Part model, mm, in its own coordinate system. A direction names the side the tool comes from. Give positions to 0.01 mm unless a question says otherwise; leave off trailing zeros. Order: outer loops, then holes, each group sorted by start corner. A loop starts at its lowest first (then second) coordinate and runs counter-clockwise, first axis right, second up. Notation, with made-up numbers: M -11.5,88.5 L 20.5,88.5 A18 cw 20.5,121.5 Z; hole C -38,-7.5 d4. An arc over 180 degrees is marked long. Return JSON: item names as keys, results as strings.
from build123d import *

# Parameters (mm, degrees)
SKETCH1_W           = 45
SKETCH1_H           = 55
BOSS_EXTRUDE1_DEPTH = 165
BOSS_EXTRUDE2_DEPTH = 75
SKETCH3_W           = 205
SKETCH3_H           = 80
CUT_EXTRUDE1_DEPTH  = 5
SKETCH4_W           = 205
SKETCH4_H           = 70
CUT_EXTRUDE2_DEPTH  = 15


with BuildPart() as part:
    # Sketch1 → Boss-Extrude1 (new body)
    with BuildSketch(Plane.XY):
        with Locations((22.5, 27.5)):
            Rectangle(SKETCH1_W, SKETCH1_H)
    extrude(amount=BOSS_EXTRUDE1_DEPTH)

    # Sketch2 → Boss-Extrude2 (add)
    with BuildSketch(Plane(origin=(0, 0, 0), x_dir=(-1, 0, 0), z_dir=(0, 0, -1))):
        Polygon((0, 0), (80, 0), (80, 80), (-125, 80), (-125, 0), (-45, 0), align=None)
    extrude(amount=-BOSS_EXTRUDE2_DEPTH)

    # Sketch3 → Cut-Extrude1 (cut)
    with BuildSketch(Plane(origin=(0, 0, 0), x_dir=(-1, 0, 0), z_dir=(0, 0, -1))):
        with Locations((-22.5, 40)):
            Rectangle(SKETCH3_W, SKETCH3_H)
    extrude(amount=-CUT_EXTRUDE1_DEPTH, mode=Mode.SUBTRACT)

    # Sketch4 → Cut-Extrude2 (cut)
    with BuildSketch(Plane(origin=(0, 80, 0), x_dir=(1, 0, 0), z_dir=(0, 1, 0))):
        with Locations((22.5, -40)):
            Rectangle(SKETCH4_W, SKETCH4_H)
    extrude(amount=-CUT_EXTRUDE2_DEPTH, mode=Mode.SUBTRACT)


solid = part.part
Q1. Band-saw the part on B-B (x = 27). Give the cut face in (y, z).
Established:
{"outline": "M 0,5 L 65,5 L 65,75 L 55,75 L 55,165 L 0,165 Z"}
Q2. Band-saw the part on D-D (x = 64). Give the cut face in (y, z).
Established:
{"outline": "M 0,5 L 65,5 L 65,75 L 0,75 Z"}
Q3. Band-saw the part on C-C (z = 153). Give the cut face in (x, y), then the cut area to 4 significant figures.
Established:
{"outline": "M 0,0 L 45,0 L 45,55 L 0,55 Z", "area": "2,475 mm²"}
Q4. 3-axis set-ups, long thin cutter, end or side, ignore diameter. For faces 1 (the flat face through (125, 33, 40)), 2 (the flat face through (24, 0, 48)), 3 (the flat face through (45, 27, 119)), 4 (the flat face through (22, 55, 119)), 5 (the flat face through (0, 27, 119)): which of +Z, -Z, +X, -X, +Y, -Y reach the whole face in a straight line?
Established:
{"face 1": "+Z, -Z, +X, +Y, -Y", "face 2": "+Z, -Z, +X, -X, -Y", "face 3": "+Z, +X, +Y, -Y", "face 4": "+Z, +X, -X, +Y", "face 5": "+Z, -X, +Y, -Y"}
Q5. Band-saw the part on A-A (y = 32). Give the cut face in (x, z).
Established:
{"outline": "M -80,5 L 125,5 L 125,75 L 45,75 L 45,165 L 0,165 L 0,75 L -80,75 Z"}
Q6. Probe line 1 along Z through (x, y) = (-17, 33.5); line 2 along X through (y, z) = (7, 131.5). List the from-to ranges inside material, lowest first.
Established:
{"line 1": "z = 5 to 75", "line 2": "x = 0 to 45"}
Q7. Pin check, flat tips, straight feed: pin 1 (1.5 mm diameter, centred on y = 14.5, z = 143.5, fed in from -X); pin 2 (1.5 mm diameter, centred on y = 44.5, z = 114.5, fed in from +X). Stop position of each tip, or through.
Established:
{"pin 1": "stops at x = 0", "pin 2": "stops at x = 45"}
